```python
from build123d import *

# Parameters (mm, degrees)
SKETCH1_W           = 150
SKETCH1_H           = 100
BOSS_EXTRUDE1_DEPTH = 3
SKETCH2_W           = 12
SKETCH2_H           = 6
BOSS_EXTRUDE2_DEPTH = 12
SKETCH4_R           = 1.625
CUT_EXTRUDE1_DEPTH  = 181.676506497
SKETCH5_W           = 13
SKETCH5_H           = 100
CUT_EXTRUDE2_DEPTH  = 181.900525151


with BuildPart() as part:
    # Sketch1 → Boss-Extrude1 (new body)
    with BuildSketch(Plane(origin=(0, 0, 0), x_dir=(1, 0, 0), z_dir=(0, 1, 0))):
        with Locations((75, 50)):
            Rectangle(SKETCH1_W, SKETCH1_H)
    extrude(amount=BOSS_EXTRUDE1_DEPTH)

    # Sketch2 → Boss-Extrude2 (add)
    with BuildSketch(Plane.XZ):
        with Locations((6, -3)):
            Rectangle(SKETCH2_W, SKETCH2_H)
        with Locations((144, -3)):
            Rectangle(SKETCH2_W, SKETCH2_H)
        with Locations((144, -97)):
            Rectangle(SKETCH2_W, SKETCH2_H)
        with Locations((6, -97)):
            Rectangle(SKETCH2_W, SKETCH2_H)
    extrude(amount=BOSS_EXTRUDE2_DEPTH)

    # Sketch4 → Cut-Extrude1 (cut, through all)
    with BuildSketch(Plane.XY):
        with Locations((6, -6)):
            Circle(SKETCH4_R)
        with Locations(Location((144, -6, 0), (0, 0, 180))):
            Circle(SKETCH4_R)
    extrude(amount=-CUT_EXTRUDE1_DEPTH, mode=Mode.SUBTRACT)

    # Sketch5 → Cut-Extrude2 (cut, through all)
    with BuildSketch(Plane(origin=(0, 3, 0), x_dir=(1, 0, 0), z_dir=(0, 1, 0))):
        with Locations((143.5, 50)):
            Rectangle(SKETCH5_W, SKETCH5_H)
    extrude(amount=-CUT_EXTRUDE2_DEPTH, mode=Mode.SUBTRACT)


solid = part.part
```
Source: CAD feature listing. Evaluate the final solid. Frame: model axes, mm. A direction names the side the tool comes from. Round coordinates to 2 decimals unless told otherwise and drop trailing zeros. Loops run counter-clockwise (first coordinate to the right, second up) from the corner with the lowest first, then second, coordinate; pieces in that order, holes last.
1. Access query for faces 1 (the flat face through (4.6, -4.6, -6)), 2 (the flat face through (6, -12, -3)), 3 (the flat face through (12, -6, -3)). Directions: +Z, -Z, +X, -X, +Y, -Y. A direction counts if a zero-diameter tool reaches every point of the face in a straight line with its end or side. Return the directions, or none.
2. Section query A-A on x = 6. Output: boundary loops of the cut face in (y, z) (3 decimals).
3. Contact query for flat-ended pins moving along their axis: pin 1 (8 mm diameter, centred on x = 65.5, z = -84, fed in from -Y); pin 2 (1.8 mm diameter, centred on y = -4.5, z = -98.5, fed in from +X). Output: stop coordinate, or through.
4. Section query D-D on z = -65. Output: boundary loops of the cut face in (x, y), and give its area (3 significant figures).
5. Section query C-C on x = 101.5. Output: boundary loops of the cut face in (y, z).
6. Ray query, L1, parallel to Y at x = 6, z = -97 (3 decimals); L2, parallel to Y at x = 82, z = -86; L3, parallel to X at y = -3, z = -95. Return the intervals inside material, ascending.
7. Mould query, pull axis X, two halves, no side actions, for faces 4 (the flat face through (68, 3, -51)), 5 (the flat face through (137, 2, -49)), 6 (the cylindrical face through (4.802, -4.902, -96.958)). Classes: released by +X, released by -X, zero draft, split by the parting line, or undercut.
8. Section query B-B on y = -2.5. Output: boundary loops of the cut face in (x, z), and give its area (3 significant figures).
Answers below:
1. face 1: +X, -X, -Y
1. face 2: +Z, -Z, +X, -X, -Y
1. face 3: +Z, -Z, +X, -Y
2. outline: (-12, -100) - (-7.625, -100) - (-7.625, -94) - (-12, -94) - close; (-12, -6) - (-7.625, -6) - (-7.625, 0) - (-12, 0) - close; (-4.375, -100) - (3, -100) - (3, 0) - (-4.375, 0) - (-4.375, -6) - (0, -6) - (0, -94) - (-4.375, -94) - close
3. pin 1: stops at y = 0
3. pin 2: stops at x = 12
4. outline: (0, 0) - (137, 0) - (137, 3) - (0, 3) - close
4. area: 411 mm2
5. outline: (0, -100) - (3, -100) - (3, 0) - (0, 0) - close
6. L1: y = -12 to -7.625, -4.375 to 3
6. L2: y = 0 to 3
6. L3: x = 0 to 12
7. face 4: zero draft
7. face 5: released by +X
7. face 6: undercut
8. outline: (0, -100) - (12, -100) - (12, -94) - (0, -94) - close; (0, -6) - (12, -6) - (12, 0) - (0, 0) - close
8. area: 144 mm2
